Part model, mm, in its own coordinate system. A direction names the side the tool comes from. Give positions to 0.01 mm unless a question says otherwise; leave off trailing zeros. Order: outer loops, then holes, each group sorted by start corner. A loop starts at its lowest first (then second) coordinate and runs counter-clockwise, first axis right, second up. Notation, with made-up numbers: M 12.25,61 L 64.25,61 A15 cw 64.25,73 Z; hole C 72,15.5 d5. An arc over 180 degrees is marked long. Return JSON: item names as keys, results as strings.
from build123d import *

# Parameters (mm, degrees)
SKETCH1_R           = 33.5
BOSS_EXTRUDE1_DEPTH = 32
CHAMFER1_SIZE       = 3
SKETCH2_W           = 62
SKETCH2_H           = 20
CUT_EXTRUDE1_DEPTH  = 25
SKETCH3_R           = 6
CUT_EXTRUDE2_DEPTH  = 40
CIRPATTERN1_COUNT   = 3


with BuildPart() as part:
    # Sketch1 → Boss-Extrude1 (new body)
    with BuildSketch(Plane(origin=(0, 0, 0), x_dir=(1, 0, 0), z_dir=(0, 1, 0))):
        with BuildLine():
            ThreePointArc((17.5, 80), (55.889587347, 32.2678683), (78.032032303, -24.844555434))
            ThreePointArc((78.032032303, -24.844555434), (72.020850643, -41.581257506), (60.532032303, -55.155444566))
            ThreePointArc((60.532032303, -55.155444566), (0, -64.5357366), (-60.532032303, -55.155444566))
            ThreePointArc((-60.532032303, -55.155444566), (-72.020850643, -41.581257506), (-78.032032303, -24.844555434))
            ThreePointArc((-78.032032303, -24.844555434), (-55.889587347, 32.2678683), (-17.5, 80))
            ThreePointArc((-17.5, 80), (0, 83.162515012), (17.5, 80))
        make_face()
        with Locations(Location((0, 0, 0), (0, 0, 270))):
            Circle(SKETCH1_R, mode=Mode.SUBTRACT)
    extrude(amount=BOSS_EXTRUDE1_DEPTH)

    # Chamfer1
    chamfer1_edges = [part.edges().sort_by_distance(p)[0] for p in [
        (0, 32, -33.5),
    ]]
    chamfer(chamfer1_edges, length=CHAMFER1_SIZE)

    # Sketch2 → Cut-Extrude1 (cut)
    with BuildSketch(Plane.XZ):
        with Locations((0, 55)):
            Rectangle(SKETCH2_W, SKETCH2_H)
    cut_extrude1 = extrude(amount=-CUT_EXTRUDE1_DEPTH, mode=Mode.SUBTRACT)

    # Sketch3 → Cut-Extrude2 (cut, symmetric)
    with BuildSketch(Plane(origin=(0, 0, 0), x_dir=(0, 0, -1), z_dir=(1, 0, 0))):
        with Locations(Location((-53.559315298, 12.5, 0), (0, 0, 180))):
            Circle(SKETCH3_R)
    cut_extrude2 = extrude(amount=CUT_EXTRUDE2_DEPTH, both=True, mode=Mode.SUBTRACT)

    # CirPattern1: Cut-Extrude1, Cut-Extrude2 ×3 about axis
    cirpattern1_axis = Axis((0, 0, 0), (0, 1, 0))
    add([cut_extrude1.rotate(cirpattern1_axis, i * 360 / CIRPATTERN1_COUNT) for i in range(1, CIRPATTERN1_COUNT)], mode=Mode.SUBTRACT)
    add([cut_extrude2.rotate(cirpattern1_axis, i * 360 / CIRPATTERN1_COUNT) for i in range(1, CIRPATTERN1_COUNT)], mode=Mode.SUBTRACT)


solid = part.part
Q1. Pin check, flat tips, straight feed: pin 1 (1.5 mm diameter, centred on y = 8.5, z = 38.5, fed in from +X); pin 2 (8.5 mm diameter, centred on y = 6.5, z = 58, fed in from -X); pin 3 (15.5 mm diameter, centred on y = 12.5, z = 53.56, fed in from -X). Stop position of each tip, or through.
Established:
{"pin 1": "stops at x = 74.02", "pin 2": "stops at x = -62.16", "pin 3": "stops at x = -69.29"}
Q2. Band-saw the part on A-A (x = 0). Give the cut face in (y, z).
Established:
{"outline": "M 0,-83.16 L 32,-83.16 L 32,-36.5 L 29,-33.5 L 0,-33.5 Z; M 0,33.5 L 29,33.5 L 32,36.5 L 32,64.54 L 25,64.54 L 25,45 L 0,45 Z"}
Q3. Two-plate mould, pull along Y, no slides. Class faces 1 (the flat face through (-66.722, 9.547, -2.726)), 2 (the flat face through (-66.311, 12.416, 7.903)), 3 (the flat face through (36, 0, 5)): +Y half, -Y half, draft (parallel to the pull), parting line (faces both ways), or undercut.
Established:
{"face 1": "draft", "face 2": "undercut", "face 3": "-Y half"}
Q4. Probe line 1 along X through (y, z) = (22, 0); line 2 along Z through (x, y) = (-1, 22); line 3 along Z through (x, y) = (-37.25, 12.5). List the from-to ranges inside material, lowest first.
Established:
{"line 1": "x = -70.87 to -62, -51.96 to -33.5, 33.5 to 51.96, 62 to 70.87", "line 2": "z = -83.15 to -33.49, 33.49 to 45", "line 3": "z = -59.19 to -57.3, -25.48 to 47.56, 59.56 to 61.04"}
Q5. 3-axis set-ups, long thin cutter, end or side, ignore diameter. For faces 4 (the flat face through (-35.72, 9.55, -56.42)), 5 (the flat face through (0, 12, 45)), 6 (the flat face through (-26.31, 12.42, -61.38)), 7 (the flat face through (35.72, 9.55, -56.42)): which of +Z, -Z, +X, -X, +Y, -Y reach the whole face in a straight line?
Established:
{"face 4": "-X, -Y", "face 5": "+Z, -Y", "face 6": "none", "face 7": "+X, -Y"}
Q6. Band-saw the part on C-C (z = -47). Give the cut face in (x, y).
Established:
{"outline": "M -46.5,25 L -24.83,25 L -24.83,0 L 24.83,0 L 24.83,25 L 46.5,25 L 46.5,32 L -46.5,32 Z"}
Q7. Band-saw the part on D-D (z = 40). Give the cut face in (x, y).
Established:
{"outline": "M -72.9,0 L 72.9,0 L 72.9,32 L -72.9,32 Z"}
Q8. Band-saw the part on B-B (y = 21). Give the cut face in (x, z).
Established:
{"outline": "M -78.03,24.84 A200 ccw -69.3,-4.21 L -54.47,4.35 L -23.47,-49.35 L -38.3,-57.91 A200 ccw -17.5,-80 A50 ccw 17.5,-80 A200 ccw 38.3,-57.91 L 23.47,-49.35 L 54.47,4.35 L 69.3,-4.21 A200 ccw 78.03,24.84 A50 ccw 60.53,55.16 A200 ccw 31,62.12 L 31,45 L -31,45 L -31,62.12 A200 ccw -60.53,55.16 A50 ccw Z; hole C 0,0 d67"}
